Build history of the part. All positions in model axes, mm. A direction names the side the tool comes from. Round coordinates to 2 decimals unless told otherwise and drop trailing zeros. Loops run counter-clockwise (first coordinate to the right, second up) from the corner with the lowest first, then second, coordinate; pieces in that order, holes last.
from build123d import *

# Parameters (mm, degrees)
F1_DEPTH = 5.5
F2_W     = 1.747264
F2_H     = 0.5
F2_W_2   = 2.660204
F3_DEPTH = 25
F4_W     = 3.051504
F4_H     = 1.634434
F5_DEPTH = 0.5
F6_R     = 0.613882
F6_W     = 0.346699
F6_H     = 1.139151
F6_W_2   = 1.22809
F6_H_2   = 0.341659
F7_DEPTH = 0.25
F9_DEPTH = 0.125
F10_R    = 0.1


with BuildPart() as f1:
    # F0 (on Front) → F1 (new body)
    with BuildSketch(Plane.XZ):
        Polygon((-7.807526, 2.338965), (-12.75, 0), (-11.363133, -1.99297), (-6.944289, -1.99297), (-6.944289, -3.057505), (-3.40048, -3.057505), (-3.40048, -8.799218), (3.6498, -8.777764), (3.63288, -3.217265), (7.91198, -3.204243), (8.126297, -3.204243), (8.126297, -1.036535), (12.75, -1.022465), (12.75, 2.348977), (7.918047, 2.334274), (7.91198, 4.327958), (7.910354, 4.862492), (6.47919, 4.862492), (-7.807526, 4.862492), (-7.807526, 3.205703), align=None)
    extrude(amount=F1_DEPTH)

    # F2 (on face) → F3 (cut)
    with BuildSketch(Plane.XY.offset(4.862492)):
        with Locations((-6.933894, -0.25)):
            Rectangle(F2_W, F2_H)
        with Locations((-6.477424, -5.25)):
            Rectangle(F2_W_2, F2_H)
    extrude(amount=-F3_DEPTH, mode=Mode.SUBTRACT)

    # F4 (on face) → F5 (cut)
    with BuildSketch(Plane.XZ.offset(5.5)):
        with Locations((-3.62157, 3.023124)):
            Rectangle(F4_W, F4_H)
    extrude(amount=-F5_DEPTH, mode=Mode.SUBTRACT)

    # F6 (on face) → F7 (join)
    with BuildSketch(Plane.XZ.offset(5)):
        with Locations((-6.103006, 2.588122)):
            Circle(F6_R)
        with Locations((-6.90784, 2.57574)):
            Rectangle(F6_W, F6_H)
        with Locations((-5.761367, 4.522246)):
            Rectangle(F6_W_2, F6_H_2)
    extrude(amount=F7_DEPTH)

    # F8 (on face) → F9 (join)
    with BuildSketch(Plane.XZ.offset(5.5)):
        Polygon((-4.826936, 3.937273), (-4.682599, 3.937712), (-4.610811, 4.062931), (-4.68336, 4.187711), (-4.827697, 4.187272), (-4.899485, 4.062053), align=None)
        Polygon((-4.827317, 1.687492), (-4.682979, 1.687492), (-4.61081, 1.812492), (-4.682979, 1.937492), (-4.827317, 1.937492), (-4.899485, 1.812492), align=None)
    extrude(amount=F9_DEPTH)

    # F10
    f10_edges = [f1.edges().sort_by_distance(p)[0] for p in [
        (-4.863591, -5.625, 4.124663),
        (-4.86321, -5.625, 3.999663),
        (-4.754767, -5.625, 3.937493),
        (-4.647085, -5.625, 4.125321),
        (-4.755528, -5.625, 4.187492),
        (-4.646705, -5.625, 4.000322),
        (-4.755148, -5.625, 1.937492),
        (-4.646895, -5.625, 1.874992),
        (-4.646895, -5.625, 1.749992),
        (-4.755148, -5.625, 1.687492),
        (-4.863401, -5.625, 1.749992),
        (-4.863401, -5.625, 1.874992),
    ]]
    fillet(f10_edges, radius=F10_R)


solid = f1.part
(1) Pull direction X, two halves, no side cores. Call faces 4 (the face through (-10, -5.5, 0)), 5 (the face through (-6.944, -2.7, -2.5)), 6 (the face through (-6, -5, 1)), 7 (the face through (-7, -0.5, 1)): +X half, -X half, draft (parallel to the pull), parting line (faces both ways), or undercut.
Responses:
face 4: draft
face 5: -X half
face 6: undercut
face 7: undercut
(2) Slice it at B-B on z = -1.5. List the corners of the cut face in (x, y), plus the area to 3 significant figures.
Responses:
outline: (-11.71, -5.5) - (-7.81, -5.5) - (-7.81, -5) - (-5.15, -5) - (-5.15, -5.5) - (8.13, -5.5) - (8.13, 0) - (-6.06, 0) - (-6.06, -0.5) - (-7.81, -0.5) - (-7.81, 0) - (-11.71, 0) - close
area: 107 mm2
(3) Slice it at C-C on x = -3. List the corners of the cut face in (y, z), plus the area to 3 significant figures.
Responses:
outline: (-5.5, -8.8) - (0, -8.8) - (0, 4.86) - (-5.5, 4.86) - (-5.5, 3.84) - (-5, 3.84) - (-5, 2.21) - (-5.5, 2.21) - close
area: 74.3 mm2
(4) Slice it at D-D on z = 1. List the corners of the cut face in (x, y), plus the area to 3 significant figures.
Responses:
outline: (-10.64, -5.5) - (-7.81, -5.5) - (-7.81, -5) - (-5.15, -5) - (-5.15, -5.5) - (12.75, -5.5) - (12.75, 0) - (-6.06, 0) - (-6.06, -0.5) - (-7.81, -0.5) - (-7.81, 0) - (-10.64, 0) - close
area: 126 mm2
(5) Pin check, flat tips, straight feed: P1, Ø3, axis at x = 6, z = -7, coming from the -Y side; P2, Ø1.5, axis at y = -4.5, z = -1, coming from the -X side; P3, Ø1.7, axis at x = -4, z = 1, coming from the -Y side; P4, Ø3, axis at x = 3, y = -2, coming from the -Z side. Stop position of each tip, or through.
Responses:
P1: passes through
P2: stops at x = -12.58
P3: stops at y = -5.5
P4: stops at z = -8.78
(6) Slice it at A-A on y = -2.05. List the corners of the cut face in (x, z).
Responses:
outline: (-12.75, 0) - (-11.36, -1.99) - (-6.94, -1.99) - (-6.94, -3.06) - (-3.4, -3.06) - (-3.4, -8.8) - (3.65, -8.78) - (3.63, -3.22) - (7.91, -3.2) - (8.13, -3.2) - (8.13, -1.04) - (12.75, -1.02) - (12.75, 2.35) - (7.92, 2.33) - (7.91, 4.33) - (7.91, 4.86) - (-7.81, 4.86) - (-7.81, 2.34) - close
(7) Which spindle directions (+Z, -Z, +X, -X, +Y, -Y) get a long thin tool onto all of the face, cutting with end or side? Do faces 1 (the face through (-7.808, -3, 4)), 2 (the face through (-6, -5.25, 3)), 3 (the face through (-3.4, -3, -6)). Say none if no direction does.
Responses:
face 1: +Z, -X, +Y, -Y
face 2: +Z, -Z, -Y
face 3: -Z, -X, +Y, -Y
(8) Probe line 1 (Z direction, x = -4.25, y = -5.35); line 2 (Y direction, x = 1.25, z = -6); line 3 (X direction, y = -0.35, z = 2.75). List the from-to ranges inside material, lowest first.
Responses:
line 1: z = -3.06 to 2.21, 3.84 to 4.86
line 2: y = -5.5 to 0
line 3: x = -6.06 to 7.92
